The drawing under review shows one solid part. Ordinate dimensions are in mm from its lowest x, y, z. A direction names the side the tool comes from. Coordinates: 2 decimals unless noted, no trailing zeros. Write each loop counter-clockwise with the first axis right and the second up, starting at its lowest first coordinate (ties: lowest second). Pieces come first, ordered by that corner, then holes. Notation, with made-up numbers: (74, -17.75) - (98, -17.75) arc R11 ccw to (98, -3.75) - close; hole circle Ø5 at (-11, 30). An arc over 180 degrees is marked (long way). Put each result on its own line as item: value. Start each with the question number.
Item 1: Machinability: for the marked faces 4 and 5, which of the approach directions +Z, -Z, +X, -X, +Y, -Y give a long, thin tool a straight path to every point of the face, cutting with its end or side? Answer none if there is none.
Item 2: Consider section B-B on y = 1.25. Give the boundary of the cut face in (x, z).
Item 3: To check wall thickness, follow L1, parallel to X at y = 0.9, z = 2.75; L2, parallel to Z at x = 13.5, y = 1.2. State the ranges of each line that lie inside material, in increasing order. Write a range as [from, to].
Item 4: For pin 1 (10 mm diameter, centred on x = 5, z = 22, fed in from -Y); pin 2 (3.5 mm diameter, centred on x = 13.5, z = 2.75, fed in from +Y); pin 3 (4 mm diameter, centred on x = 16.5, z = 24, fed in from +Y); pin 4 (8 mm diameter, centred on x = 20.5, z = 21, fed in from +Y), all flat-tipped, find the tip position at first contact; note any pin that passes through.
Item 5: Consider section A-A on x = 13.5. Give the boundary of the cut face in (y, z), then the cut area to 3 significant figures.
Item 6: Consider section C-C on z = 38. Give the boundary of the cut face in (x, y).
Item 7: Mouldability with a two-part tool opening along Z and no side actions: class the marked faces 1, 2 and 3 as pulls with the +Z half, pulls with the -Z half, needs draft (parallel to the pull), parting line crosses it, or undercut.
Item 8: Consider section D-D on y = 5.25. Give the boundary of the cut face in (x, z).
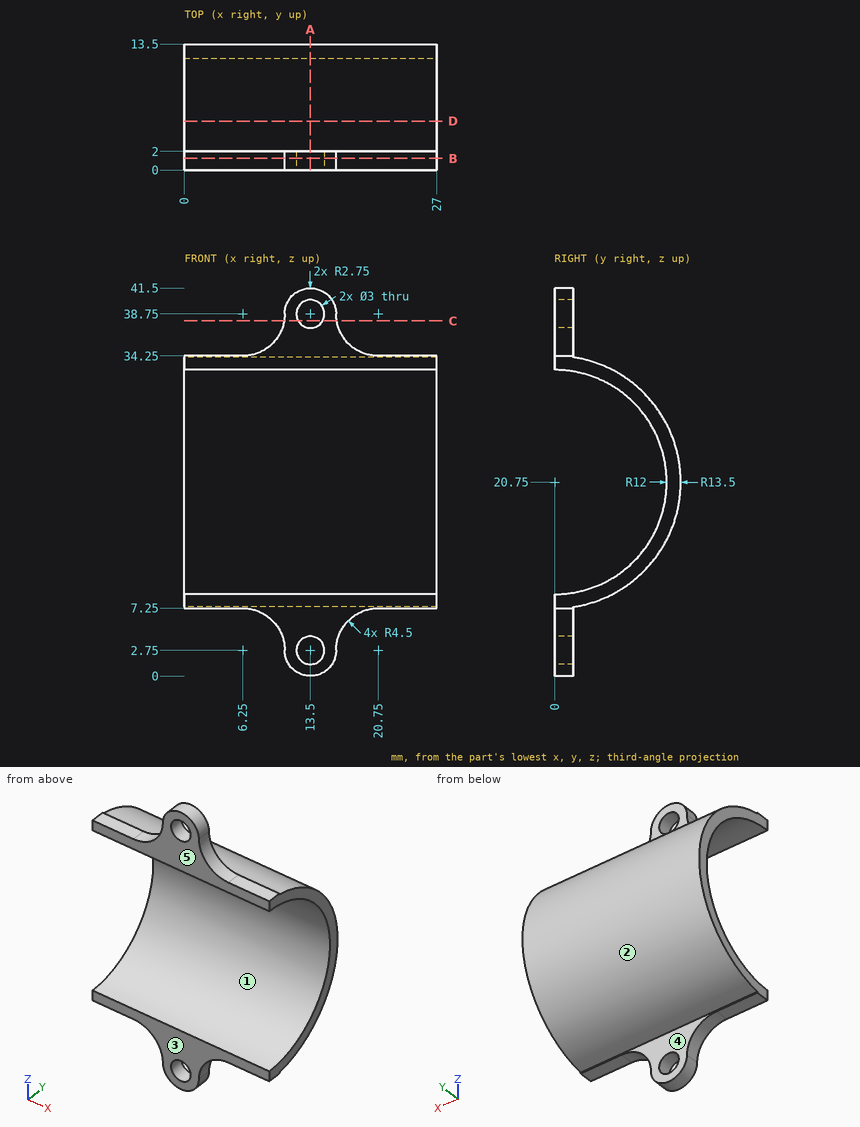
Report:
1. face 4: -Z, +X, -X, +Y
1. face 5: +Z, -Z, +X, -X, -Y
2. outline: (0, 7.25) - (6.25, 7.25) arc R4.5 cw to (10.75, 2.75) arc R2.75 ccw to (16.25, 2.75) arc R4.5 cw to (20.75, 7.25) - (27, 7.25) - (27, 8.82) - (0, 8.82) - close; (0, 32.68) - (27, 32.68) - (27, 34.25) - (20.75, 34.25) arc R4.5 cw to (16.25, 38.75) arc R2.75 ccw to (10.75, 38.75) arc R4.5 cw to (6.25, 34.25) - (0, 34.25) - close; hole circle Ø3 at (13.5, 2.75); hole circle Ø3 at (13.5, 38.75)
3. L1: [10.75, 12], [15, 16.25]
3. L2: [0, 1.25], [4.25, 8.81], [32.69, 37.25], [40.25, 41.5]
4. pin 1: y = 10.24
4. pin 2: y = 2
4. pin 3: y = 13.44
4. pin 4: y = 13.5
5. outline: (0, 0) - (2, 0) - (2, 1.25) - (0, 1.25) - close; (0, 4.25) - (2, 4.25) - (2, 7.4) arc R13.5 ccw to (2, 34.1) - (2, 37.25) - (0, 37.25) - (0, 32.75) arc R12 cw to (0, 8.75) - close; (0, 40.25) - (2, 40.25) - (2, 41.5) - (0, 41.5) - close
5. area: 77.3 mm²
6. outline: (10.69, 0) - (12.2, 0) - (12.2, 2) - (10.69, 2) - close; (14.8, 0) - (16.31, 0) - (16.31, 2) - (14.8, 2) - close
7. face 1: undercut
7. face 2: parting line crosses it
7. face 3: needs draft
8. outline: (0, 8.31) - (27, 8.31) - (27, 9.96) - (0, 9.96) - close; (0, 31.54) - (27, 31.54) - (27, 33.19) - (0, 33.19) - close
